Build history of the part. All positions in model axes, mm. Round coordinates to 2 decimals unless told otherwise and drop trailing zeros. Write each loop counter-clockwise with the first axis right and the second up, starting at its lowest first coordinate (ties: lowest second). Pieces come first, ordered by that corner, then holes. Notation, with made-up numbers: M -20,72.5 L 32,72.5 A35 ccw 32,105.5 Z; hole C -3,35.5 d3. An arc over 180 degrees is marked long. Use a Markdown table: item, result.
from build123d import *

# Parameters (mm, degrees)
SKETCH1_R           = 6
BOSS_EXTRUDE1_DEPTH = 2
FILLET1_R           = 1


with BuildPart() as part:
    # Sketch1 → Boss-Extrude1 (new body)
    with BuildSketch(Plane(origin=(0, 0, 0), x_dir=(1, 0, 0), z_dir=(0, 1, 0))):
        Polygon((7.966349656, 4.676602025), (-0.066881329, 9.23736219), (-8.033230985, 4.560760165), (-7.966349656, -4.676602025), (0.066881329, -9.23736219), (8.033230985, -4.560760165), align=None)
        Circle(SKETCH1_R, mode=Mode.SUBTRACT)
    extrude(amount=BOSS_EXTRUDE1_DEPTH)

    # Fillet1
    fillet1_edges = [part.edges().sort_by_distance(p)[0] for p in [
        (8.033230985, 1, 4.560760165),
        (0.066881329, 1, 9.23736219),
        (-7.966349656, 1, 4.676602025),
        (-8.033230985, 1, -4.560760165),
        (-0.066881329, 1, -9.23736219),
        (7.966349656, 1, -4.676602025),
    ]]
    fillet(fillet1_edges, radius=FILLET1_R)


solid = part.part
Q1. Cut at B-B on x = -3. Give the cut face in (y, z).
Response values:
| item | result |
|---|---|
| outline | M 0,-7.52 L 2,-7.52 L 2,-5.2 L 0,-5.2 Z; M 0,5.2 L 2,5.2 L 2,7.5 L 0,7.5 Z |
Q2. Cut at A-A on y = 1.7. Give the cut face in (x, z), and give its area (3 significant figures).
Response values:
| item | result |
|---|---|
| outline | M -8.03,-3.98 A1 ccw -7.54,-4.85 L -0.56,-8.95 A1 ccw 0.44,-8.95 L 7.46,-4.96 A1 ccw 7.97,-4.1 L 8.03,3.98 A1 ccw 7.54,4.85 L 0.56,8.95 A1 ccw -0.44,8.95 L -7.46,4.96 A1 ccw -7.97,4.1 Z; hole C 0,0 d12 |
| area | 108 mm2 |
Q3. Drill centre lines: L1, parallel to Z at x = 0, y = 1.2; L2, parallel to X at y = 0.45, z = 0.25; L3, parallel to Z at x = 1.75, y = 0.95. Where is each one in solid material? Low to high.
Response values:
| item | result |
|---|---|
| L1 | z = -9.08 to -6, 6 to 9.08 |
| L2 | x = -8 to -5.99, 5.99 to 8 |
| L3 | z = -8.21 to -5.74, 5.74 to 8.25 |
Q4. Cut at D-D on z = -7. Give the cut face in (x, y), and give its area (3 significant figures).
Response values:
| item | result |
|---|---|
| outline | M -3.88,0 L 3.87,0 L 3.87,2 L -3.88,2 Z |
| area | 15.5 mm2 |
Q5. Cut at C-C on z = 0. Give the cut face in (x, y), and give its area (3 significant figures).
Response values:
| item | result |
|---|---|
| outline | M -8,0 L -6,0 L -6,2 L -8,2 Z; M 6,0 L 8,0 L 8,2 L 6,2 Z |
| area | 8.00 mm2 |
Q6. Two-plate mould, pull along X, no slides. Class faces 1 (the flat face through (2, 0, 6)), 2 (the cylindrical face through (7.9, 1.01, 4.48)), 3 (the cylindrical face through (-6, 1, 0)): +X half, -X half, draft (parallel to the pull), parting line (faces both ways), or undercut.
Response values:
| item | result |
|---|---|
| face 1 | draft |
| face 2 | +X half |
| face 3 | undercut |
Q7. Drop a flat-ended pin along its axis: P1, Ø1, axis at y = 1, z = -2, coming from the -X side. Give the stop position or say it passes through.
Response values:
| item | result |
|---|---|
| P1 | stops at x = -8.02 |
